Autodesk Inventor part; units mm, degrees
ref_plane "XZ Plane" through (0, 0, 0) normal (0, 1, 0) x (-1, 0, 0)
ref_plane "XY Plane" through (0, 0, 0) normal (0, 0, 1) x (1, 0, 0)
sketch "Sketch1" plane through (0, 0, 0) normal (0, 0, 1) x (1, 0, 0)
  line L0 (0, 17.78) -> (0, -17.78)
  line L1 (-26.67, 0) -> (26.67, 0)
  line L2 (19.05, -12.7) -> (-19.05, -12.7)
  line L3 (-19.05, -12.7) -> (-19.05, 12.7)
  line L4 (-19.05, 12.7) -> (19.05, 12.7)
  line L5 (19.05, 12.7) -> (19.05, -12.7)
  line L6 (19.05, -12.7) -> (-19.05, 12.7) construction
  line L7 (-19.05, -12.7) -> (19.05, 12.7) construction
  point P0 (0, 0)
  dimension "d0" = 25.4
  dimension "d1" = 38.1
extrude "Extrusion1" add sketch "Sketch1" along normal blind 6.35
sketch "Sketch2" plane through (0, 0, 0) normal (0, 0, 1) x (1, 0, 0)
  line L0 (0, 13.335) -> (0, -13.335)
  line L1 (19.05, -12.7) -> (19.05, 12.7)
  line L2 (-19.05, -12.7) -> (19.05, -12.7)
  point P0 (0, 0)
  point P1 (2.54, 0)
  point P2 (-12.065, 3.175)
  dimension "d27" = 12.065
  dimension "d46" = 0
  dimension "d48" = 3.175
  dimension "d58" = 16.51
hole "Hole1" at (2.54, 0, 0) direction (0, 0, 1) diameter 4.318 end through all counterbore diameter 7.9502 counterbore depth 4.1656
sketch "Sketch3" plane through (0, 0, 0) normal (0, 0, 1) x (1, 0, 0)
  line L0 (19.05, -12.7) -> (19.05, 12.7)
  line L1 (19.05, 12.7) -> (-19.05, 12.7)
  line L2 (-19.05, -12.7) -> (19.05, -12.7)
  line L3 (0, 13.335) -> (0, -13.335)
  line L4 (-26.67, 0) -> (26.67, 0)
  line L5 (19.05, 12.7) -> (11.43, 12.7)
  line L6 (11.43, 12.7) -> (11.43, 10.16)
  line L7 (11.43, 10.16) -> (19.05, 10.16)
  line L8 (19.05, 10.16) -> (19.05, 12.7)
  line L9 (19.05, -12.7) -> (11.43, -12.7)
  line L10 (11.43, -12.7) -> (11.43, -10.16)
  line L11 (11.43, -10.16) -> (19.05, -10.16)
  line L12 (19.05, -10.16) -> (19.05, -12.7)
  point P0 (0, 0)
  dimension "d12" = 2.54
  dimension "d13" = 2.54
  dimension "d14" = 20.32
  dimension "d26" = 7.62
extrude "Extrusion2" add sketch "Sketch3" against normal blind 10.668 contours L2 L10 L11 L0 | L7 L6 L1 L0
sketch "Sketch4" plane through (-19.05, 12.7, 6.35) normal (0, 1, 0) x (1, 0, 0)
  line L0 (19.05, 20.4216) -> (19.05, -3.4036)
  line L1 (45.72, 6.35) -> (-7.62, 6.35)
  line L2 (30.48, 17.018) -> (38.1, 17.018)
  line L3 (30.48, 6.35) -> (30.48, 17.018)
  line L4 (38.1, 0) -> (38.1, 17.018)
  line L5 (38.1, 0) -> (0, 0)
  point P0 (19.05, 6.35)
  point P1 (34.29, 13.97)
  dimension "d17" = 3.81
  dimension "d18" = 3.81
  dimension "d36" = 13.97
  dimension "d62" = 3.048
hole "Hole2" at (15.24, 12.7, -7.62) direction (0, -1, 0) diameter 3.1877 end through all
hole "Hole3" [suppressed]
chamfer "Chamfer1" distance 1.905 angle 45 4 edges at (11.43, -11.43, -10.668) (19.05, -11.43, -10.668) (19.05, 11.43, -10.668) (11.43, 11.43, -10.668)
fillet "Fillet1" [suppressed]
sketch "Sketch5" plane through (0, 0, 0) normal (0, 0, -1) x (-1, 0, 0)
  line L0 (17.018, 0) -> (7.112, 0)
  line L1 (7.112, 0) -> (7.112, 6.35)
  line L2 (7.112, 6.35) -> (17.018, 6.35)
  line L3 (17.018, 6.35) -> (17.018, 0)
  line L4 (17.018, 0) -> (7.112, 6.35) construction
  line L5 (7.112, 0) -> (17.018, 6.35) construction
  line L6 (-11.43, -12.7) -> (19.05, -12.7)
  line L7 (19.05, -12.7) -> (19.05, 12.7)
  line L8 (19.05, -12.7) -> (7.62, -12.7)
  line L9 (7.62, -12.7) -> (7.62, -3.175)
  line L10 (7.62, -3.175) -> (19.05, -3.175)
  line L11 (19.05, -3.175) -> (19.05, -12.7)
  circle A0 centre (7.9057, 6.35) radius 0.7937
  circle A1 centre (16.2242, 6.35) radius 0.7937
  circle A2 centre (7.9057, 0) radius 0.7937
  circle A3 centre (16.2242, 0) radius 0.7938
  point P0 (0, 0)
  point P1 (12.065, 3.175)
  dimension "d53" = 1.5875
  dimension "d41" = 9.906
  dimension "d42" = 6.35
  dimension "d49" = 9.525
  dimension "d50" = 11.43
extrude "Extrusion3" cut sketch "Sketch5" against normal blind 1.27 contours A2 L0 | A2 L1 A0 L2 A1 L3 A3 L0 | L0 A2 | A3 L0 | L0 A3 | A0 L2 | L2 A0 | A1 L2 | L2 A1
fillet "Fillet2" [suppressed]
extrude "Extrusion4" cut sketch "Sketch5" against normal up to next contours L9 L10 L7 L6
ref_plane "Work Plane2" through (-12.065, 3.175, 0) normal (1, 0, 0) x (0, 1, 0)
fillet "Fillet3" radius 3.175 1 edges at (-7.62, -3.175, 3.175)
chamfer "Chamfer2" distance 2.54 angle 45 1 edges at (-19.05, -3.175, 3.175)
chamfer "Chamfer3" distance 2.54 angle 45 1 edges at (-19.05, 12.7, 3.175)
fillet "Fillet4" radius 3.175 1 edges at (-7.62, -12.7, 3.175)
sketch "Sketch6" plane through (0, 0, 0) normal (0, 0, 1) x (1, 0, 0)
  line L0 (0, 17.78) -> (0, -17.78)
  point P0 (0, 0)
  point P1 (-2.54, 6.985)
  point P2 (-2.54, -6.985)
  dimension "d64" = 6.985
  dimension "d65" = 13.97
  dimension "d66" = 2.54
hole "Hole4" at (-2.54, -6.985, 0) at (-2.54, 6.985, 0) direction (0, 0, 1) diameter 6.35 end through all
sketch "Sketch7" plane through (0, 0, 6.35) normal (0, 0, 1) x (1, 0, 0)
  circle A0 centre (-2.54, 6.985) radius 3.175
  circle A1 centre (-2.54, -6.985) radius 3.175
  line L0 (-1.651, 1.778) -> (-3.429, 1.778)
  line L1 (-3.429, 1.778) -> (-3.429, 12.192)
  line L2 (-3.429, 12.192) -> (-1.651, 12.192)
  line L3 (-1.651, 12.192) -> (-1.651, 1.778)
  line L4 (-1.651, 1.778) -> (-3.429, 12.192) construction
  line L5 (-3.429, 1.778) -> (-1.651, 12.192) construction
  line L6 (-3.429, -12.192) -> (-1.651, -12.192)
  line L7 (-1.651, -12.192) -> (-1.651, -1.778)
  line L8 (-1.651, -1.778) -> (-3.429, -1.778)
  line L9 (-3.429, -1.778) -> (-3.429, -12.192)
  line L10 (-3.429, -12.192) -> (-1.651, -1.778) construction
  line L11 (-1.651, -12.192) -> (-3.429, -1.778) construction
  circle A2 centre (2.54, 0) radius 2.159
  point P0 (0, 0)
  dimension "d74" = 1.778
  dimension "d75" = 10.414
  dimension "d76" = 1.778
  dimension "d77" = 10.414
extrude "Extrusion5" cut sketch "Sketch7" against normal blind 2.54 contours L3 A0 L1 | A0 L1 L2 L3 | L3 L0 L1 A0 | L7 A1 L9 | A1 L9 L8 L7 | L7 L6 L9 A1
fillet "Fillet5" radius 0.7937 8 edges at (-3.429, 12.192, 5.08) (-1.651, 12.192, 5.08) (-3.429, 1.778, 5.08) (-1.651, 1.778, 5.08) (-3.429, -1.778, 5.08) (-1.651, -1.778, 5.08) (-3.429, -12.192, 5.08) (-1.651, -12.192, 5.08)
chamfer "Chamfer4" distance 0.889 angle 45 2 edges at (-2.54, -10.16, 0) (-2.54, 3.81, 0)
properties part number "J005823" material "ALUMINUM, 6061-T651"
Source: CAD feature listing. Evaluate the final solid. Frame: model axes, mm. A direction names the side the tool comes from. Coordinates: 2 decimals unless noted, no trailing zeros. Order: outer loops, then holes, each group sorted by start corner. A loop starts at its lowest first (then second) coordinate and runs counter-clockwise, first axis right, second up. Notation, with made-up numbers: M 48,86 L 92,86 A15 ccw 92,90 Z; hole C 50.25,-38 d5. An arc over 180 degrees is marked long. Write each question's results on one line, items separated by ' | '. Start each with the question number.
1) Section query B-B (x = 15.24). Return the cut outline in (y, z).
2) Section query A-A (z = -5.25). Return the cut outline in (x, y).
3) Contact query for flat-ended pins moving along their axis: pin 1 Ø1.3 at (y, z) = (-11, -6.5) entering from -X; pin 2 Ø1.1 at (y, z) = (11, 5.5) entering from -X; pin 3 Ø2.5 at (y, z) = (-7.5, 3.5) entering from -X. Output: stop coordinate, or through.
4) Draft query along Z for faces 4 (the face through (13.66, 11.41, -7.83)), 5 (the face through (-12, 3, 1.27)), 6 (the face through (-14, -3.175, 3)). Return one class per face: released by +Z, released by -Z, zero draft, split by the parting line, or undercut.
5) Section query C-C (x = 2.54). Return the cut outline in (y, z), plus the area to 3 significant figures.
6) Section query D-D (z = 3). Return the cut outline in (x, y) (3 decimals), plus the area to 3 significant figures.
7) Access query for faces 1 (the face through (15, 10.16, -5)), 2 (the face through (-1.651, -3, 5)), 3 (the face through (-16.242, 7.144, 0.626)). Directions: +Z, -Z, +X, -X, +Y, -Y. A direction counts if a zero-diameter tool reaches every point of the face in a straight line with its end or side. Return the directions, or none.
8) Line query: line 1 (Y direction, x = -2.54, z = 2.25); line 2 (Y direction, x = -2.54, z = 5); line 3 (X direction, y = 11.3, z = -7.62). Output: solid intervals per line, ascending. Write a range as from..to.
Answers:
1) outline: M -12.7,-10.67 L -10.16,-10.67 L -10.16,-9.21 L -12.7,-9.21 Z; M -12.7,-6.03 L -10.16,-6.03 L -10.16,0 L 10.16,0 L 10.16,-6.03 L 12.7,-6.03 L 12.7,6.35 L -12.7,6.35 Z; M 10.16,-10.67 L 12.7,-10.67 L 12.7,-9.21 L 10.16,-9.21 Z
2) outline: M 11.43,-12.7 L 19.05,-12.7 L 19.05,-10.16 L 11.43,-10.16 Z; M 11.43,10.16 L 19.05,10.16 L 19.05,12.7 L 11.43,12.7 Z
3) pin 1: stops at x = 11.43 | pin 2: stops at x = -18.76 | pin 3: stops at x = -7.62
4) face 4: undercut | face 5: released by -Z | face 6: zero draft
5) outline: M -12.7,0 L -3.98,0 L -3.98,4.17 L -2.16,4.17 L -2.16,6.35 L -12.7,6.35 Z; M 2.16,4.17 L 3.98,4.17 L 3.98,0 L 12.7,0 L 12.7,6.35 L 2.16,6.35 Z | area: 119 mm^2
6) outline: M -19.05,-0.635 L -16.51,-3.175 L -10.795,-3.175 A3.175 cw -7.62,-6.35 L -7.62,-9.525 A3.175 ccw -4.445,-12.7 L 19.05,-12.7 L 19.05,12.7 L -16.51,12.7 L -19.05,10.16 Z; hole C -2.54,-6.985 d6.35; hole C -2.54,6.985 d6.35; hole C 2.54,0 d7.95 | area: 739 mm^2
7) face 1: -Z, +X, -X | face 2: +Z | face 3: -Z
8) line 1: y = -12.7..-10.16, -3.81..3.81, 10.16..12.7 | line 2: y = -12.7..-12.19, -1.78..1.78, 12.19..12.7 | line 3: x = 11.43..13.65, 16.83..19.05
